Check sheet for the modelled part. Datum: model origin and axes. Units: mm. A direction names the side the tool comes from. Give positions to 0.01 mm unless a question says otherwise; leave off trailing zeros. Order: outer loops, then holes, each group sorted by start corner. A loop starts at its lowest first (then second) coordinate and runs counter-clockwise, first axis right, second up.
from build123d import *

# Parameters (mm, degrees)
BOSS_EXTRUDE1_DEPTH  = 31.75
FILLET1_R            = 5.08
BOSS_EXTRUDE2_DEPTH  = 2.5399999999999996
SKETCH5_R            = 24.891999999999996
CUT_EXTRUDE1_DEPTH   = 2.54
SKETCH6_R            = 1.905
CUT_EXTRUDE2_DEPTH   = 80.32849774232189
LPATTERN1_COUNT      = 2
LPATTERN1_PITCH      = 55.88
LPATTERN1_COUNT_DIR2 = 2
LPATTERN1_PITCH_DIR2 = 55.88


with BuildPart() as part:
    # Sketch1 → Boss-Extrude1 (new body)
    with BuildSketch(Plane(origin=(0, 0, 0), x_dir=(1, 0, 0), z_dir=(0, 1, 0))):
        Polygon((7.620000000000001, -7.619999999999999), (-7.619999999999997, -7.620000000000001), (-7.619999999999997, 7.619999999999997), (7.62, 7.619999999999999), align=None)
    extrude(amount=BOSS_EXTRUDE1_DEPTH)

    # Fillet1
    fillet1_edges = [part.edges().sort_by_distance(p)[0] for p in [
        (-7.619999999999997, 15.875, -7.619999999999997),
        (7.62, 15.875, -7.619999999999999),
        (7.620000000000001, 15.875, 7.619999999999999),
        (-7.619999999999997, 15.875, 7.620000000000001),
    ]]
    fillet(fillet1_edges, radius=FILLET1_R)

    # Sketch3 → Revolve1 (revolve)
    with BuildSketch(Plane(origin=(0, 0, 0), x_dir=(0, 0, -1), z_dir=(1, 0, 0)), mode=Mode.PRIVATE) as revolve1_sk:
        with BuildLine():
            Line((25.00680208994189, -26.471907853088844), (27.546802089941888, -26.471907853088844))
            ThreePointArc((27.546802089941888, -26.471907853088844), (19.47853055780167, -6.993377295287178), (0, 1.0748942368530439))
            Line((0, 1.0748942368530439), (0, -1.4651057631469566))
            ThreePointArc((0, -1.4651057631469566), (17.68247933358784, -8.789428519501008), (25.00680208994189, -26.471907853088844))
        make_face()
    revolve(revolve1_sk.sketch.rotate(Axis((0, -1.26539568401347, 0), (0, -1, 0)), 180), axis=Axis((0, -1.26539568401347, 0), (0, -1, 0)))

    # Sketch4 → Boss-Extrude2 (add)
    with BuildSketch(Plane.XZ.offset(26.471907853088844)):
        Polygon((38.10000000000001, -38.099999999999994), (-38.099999999999994, -38.10000000000001), (-38.099999999999994, 38.099999999999994), (38.10000000000001, 38.10000000000001), align=None)
    extrude(amount=BOSS_EXTRUDE2_DEPTH)

    # Sketch5 → Cut-Extrude1 (cut)
    with BuildSketch(Plane.XZ.offset(29.011907853088847)):
        with Locations(Location((0, 0, 0), (0, 0, 270))):
            Circle(SKETCH5_R)
    extrude(amount=-CUT_EXTRUDE1_DEPTH, mode=Mode.SUBTRACT)

    # Sketch6 → Cut-Extrude2 (cut, through all)
    with BuildSketch(Plane(origin=(0, -26.471907853088844, 0), x_dir=(1, 0, 0), z_dir=(0, 1, 0))):
        with Locations(Location((-27.939999999999998, 27.94000000000001, 0), (0, 0, 270))):
            Circle(SKETCH6_R)
    cut_extrude2 = extrude(amount=-CUT_EXTRUDE2_DEPTH, mode=Mode.SUBTRACT)

    # LPattern1: Cut-Extrude2 2 × 2
    with Locations(*[(i * LPATTERN1_PITCH, 0, j * LPATTERN1_PITCH_DIR2) for i in range(LPATTERN1_COUNT) for j in range(LPATTERN1_COUNT_DIR2) if (i, j) != (0, 0)]):
        add(cut_extrude2, mode=Mode.SUBTRACT)


solid = part.part
1) Set-up check for faces 4 (the face through (-7.62, 16, 0)), 5 (the face through (0, 16, 7.62)), 6 (the face through (-22.08, -27.76, -11.49)), 7 (the face through (7.62, 16, 0)): record each of +Z, -Z, +X, -X, +Y, -Y from which the full face is reachable in a straight line by a thin tool's end or side.
Recorded:
face 4: +Z, -Z, -X, +Y
face 5: +Z, +X, -X, +Y
face 6: -Y
face 7: +Z, -Z, +X, +Y
2) Section check A-A, the plane y = 13. Record the cut outline in (x, z).
Recorded:
outline: (-7.62, -2.54) arc R5.08 ccw to (-2.54, -7.62) - (2.54, -7.62) arc R5.08 ccw to (7.62, -2.54) - (7.62, 2.54) arc R5.08 ccw to (2.54, 7.62) - (-2.54, 7.62) arc R5.08 ccw to (-7.62, 2.54) - close
3) Depth check by flat-ended pin: pin 1 Ø4 at (x, y) = (0.5, 11.5) entering from -Z; pin 2 Ø4 at (x, z) = (3.5, -3) entering from -Y; pin 3 Ø6 at (y, z) = (-17.5, -12.5) entering from -X; pin 4 Ø6 at (x, z) = (27.94, 27.94) entering from -Y. Enter the tip coordinate at first touch or a pass-through.
Recorded:
pin 1: stops at z = -7.62
pin 2: stops at y = -2.35
pin 3: stops at x = -24.6
pin 4: stops at y = -29.01
4) Section check B-B, the plane z = -19. Record the cut outline in (x, y).
Recorded:
outline: (-38.1, -29.01) - (-16.08, -29.01) - (-16.08, -26.47) - (-16.26, -26.47) arc R16.26 cw to (16.26, -26.47) - (16.08, -26.47) - (16.08, -29.01) - (38.1, -29.01) - (38.1, -26.47) - (19.95, -26.47) arc R19.95 ccw to (-19.95, -26.47) - (-38.1, -26.47) - close
5) Draft check along Z on faces 1 (the face through (38.1, -28, 1)), 2 (the face through (6.092, 16.097, -6.171)), 3 (the face through (-27.856, -27.724, 26.037)). Enter one of: +Z half, -Z half, draft (parallel to the pull), parting line (faces both ways), or undercut.
Recorded:
face 1: draft
face 2: -Z half
face 3: undercut
6) Material ranges on L1, parallel to X at y = -28.2, z = 27.94 (3 decimals); L2, parallel to Z at x = 27, y = -27; L3, parallel to Y at x = -9.5, z = -31.5, recorded low to high.
Recorded:
L1: x = -38.1 to -29.845, -26.035 to 26.035, 29.845 to 38.1
L2: z = -38.1 to -29.6, -26.28 to 26.28, 29.6 to 38.1
L3: y = -29.01 to -26.47
7) Section check C-C, the plane x = -9. Record the cut outline in (y, z).
Recorded:
outline: (-29.01, -38.1) - (-26.47, -38.1) - (-26.47, -26.04) arc R26.04 ccw to (-26.47, 26.04) - (-26.47, 38.1) - (-29.01, 38.1) - (-29.01, 23.21) - (-26.47, 23.21) - (-26.47, 23.33) arc R23.33 cw to (-26.47, -23.33) - (-26.47, -23.21) - (-29.01, -23.21) - close
8) Section check D-D, the plane y = -10.5. Record the cut outline in (x, z).
Recorded:
outline: circle Ø44.89 at (0, 0); hole circle Ø38.48 at (0, 0)
